Input: dimensioned drawing with shaded views. Units: mm. Origin: part minimum x, y, z. A direction names the side the tool comes from. Give positions to 0.01 mm unless a question says otherwise; leave off trailing zeros. Order: outer loops, then holes, each group sorted by start corner. A loop starts at its lowest first (then second) coordinate and runs counter-clockwise, first axis right, second up.
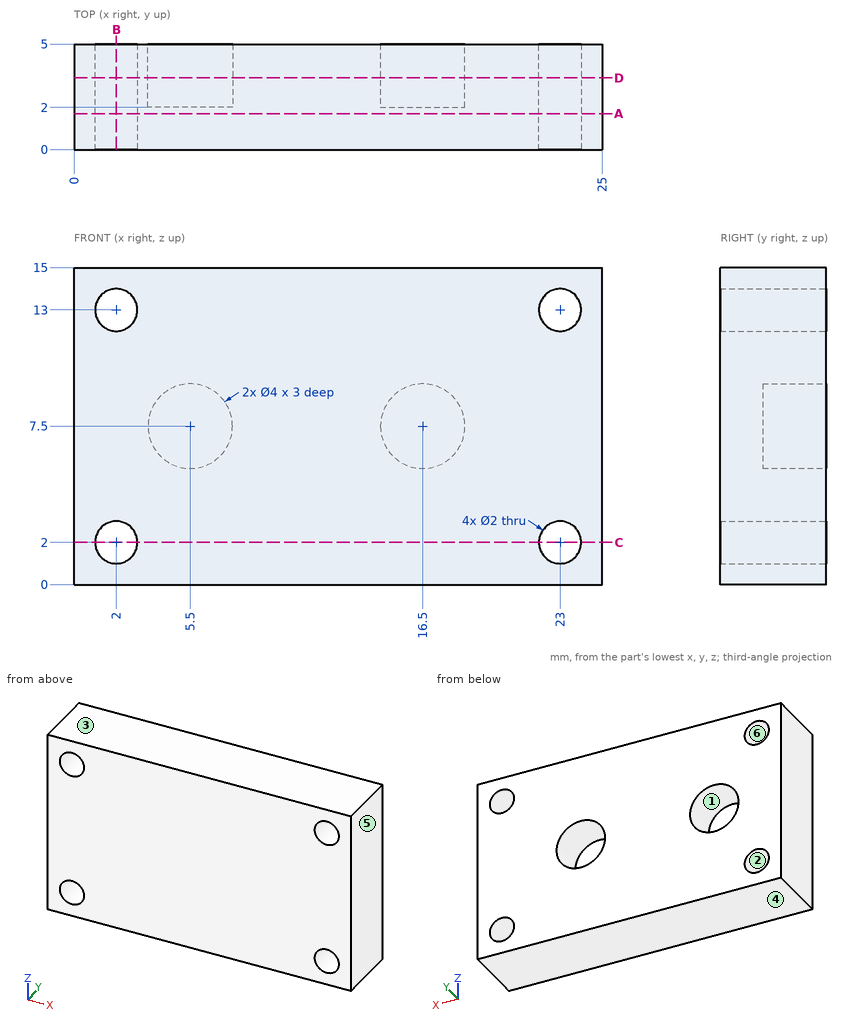
1) Section query A-A, the plane y = 1.7. Return the cut outline in (x, z).
Report:
outline: (0, 0) - (25, 0) - (25, 15) - (0, 15) - close; hole circle Ø2 at (2, 2); hole circle Ø2 at (2, 13); hole circle Ø2 at (23, 2); hole circle Ø2 at (23, 13)
2) Draft query along Z for the marked faces 3, 4, 5 and 6. Return one class per face: +Z half, -Z half, draft (parallel to the pull), parting line (faces both ways), or undercut.
Report:
face 3: +Z half
face 4: -Z half
face 5: draft
face 6: undercut
3) Pin query (flat end, axial travel): pin 1 (1.2 mm diameter, centred on x = 6.5, z = 7, fed in from +Y). Return the tip coordinate at first contact, or that it passes through.
Report:
pin 1: stops at y = 2
4) Section query D-D, the plane y = 3.4. Return the cut outline in (x, z).
Report:
outline: (0, 0) - (25, 0) - (25, 15) - (0, 15) - close; hole circle Ø2 at (2, 2); hole circle Ø2 at (2, 13); hole circle Ø4 at (5.5, 7.5); hole circle Ø4 at (16.5, 7.5); hole circle Ø2 at (23, 2); hole circle Ø2 at (23, 13)
5) Section query B-B, the plane x = 2. Return the cut outline in (y, z).
Report:
outline: (0, 0) - (5, 0) - (5, 1) - (0, 1) - close; (0, 3) - (5, 3) - (5, 12) - (0, 12) - close; (0, 14) - (5, 14) - (5, 15) - (0, 15) - close
6) Material intervals for L1, parallel to Z at x = 23, y = 1.15; L2, parallel to X at y = 1.85, z = 2.25; L3, parallel to X at y = 3.35, z = 8.25, sorted ascending.
Report:
L1: z = 0 to 1, 3 to 12, 14 to 15
L2: x = 0 to 1.03, 2.97 to 22.03, 23.97 to 25
L3: x = 0 to 3.65, 7.35 to 14.65, 18.35 to 25
7) Section query C-C, the plane z = 2. Return the cut outline in (x, y).
Report:
outline: (0, 0) - (1, 0) - (1, 5) - (0, 5) - close; (3, 0) - (22, 0) - (22, 5) - (3, 5) - close; (24, 0) - (25, 0) - (25, 5) - (24, 5) - close
8) Reachability of the marked faces 1 and 2 from +Z, -Z, +X, -X, +Y, -Y: full face, straight path, thin tool, end or side. Return the list, or none.
Report:
face 1: +Y
face 2: +Y, -Y
